Here's how the part is built. I have some questions about the finished solid (model axes, mm). Round coordinates to 2 decimals unless told otherwise and drop trailing zeros. Order: outer loops, then holes, each group sorted by start corner. A loop starts at its lowest first (then second) coordinate and runs counter-clockwise, first axis right, second up.
```python
from build123d import *

# Parameters (mm, degrees)
SKETCH1_R           = 20.32
BOSS_EXTRUDE2_DEPTH = 70.1


with BuildPart() as part:
    # Sketch1 → Boss-Extrude2 (new body)
    with BuildSketch(Plane.XY):
        with Locations((5.436965925, 8.875)):
            Circle(SKETCH1_R)
        with BuildLine():
            ThreePointArc((8.106562975, 3.61237619), (8.680765272, 1.846602096), (8.875, 0))
            ThreePointArc((8.875, 0), (-6.021266525, -6.519967365), (-0.704712549, 8.84697718))
            ThreePointArc((-0.704712549, 8.84697718), (-6.013906314, 24.19612946), (8.8646, 17.683521379))
            ThreePointArc((8.8646, 17.683521379), (8.683960375, 15.903081724), (8.149403519, 14.195204385))
            ThreePointArc((8.149403519, 14.195204385), (18.04408912, 17.284412427), (24.1046, 8.875))
            ThreePointArc((24.1046, 8.875), (18.010024125, 0.454305284), (8.106562975, 3.61237619))
        make_face(mode=Mode.SUBTRACT)
    extrude(amount=BOSS_EXTRUDE2_DEPTH)


solid = part.part
```
1) If we section it at A-A (x = 13.5): Write out the boundary of the cut face in (y, z), plus the area to 3 significant figures.
2) I'm going to push flat-ended pins straight in: pin 1 (5 mm diameter, centred on x = -7.5, z = 20, fed in from -Y); pin 2 (5 mm diameter, centred on y = 4, z = 54.5, fed in from -X); pin 3 (4 mm diameter, centred on x = 18.5, z = 17, fed in from -Y). Where does each tip first touch, or does it pass through?
3) If we section it at D-D (x = -8): Write out the boundary of the cut face in (y, z) (3 decimals), plus the area to 3 significant figures.
4) If we section it at C-C (z = 13.5): Write out the boundary of the cut face in (x, y) (3 decimals), plus the area to 3 significant figures.
5) If we section it at B-B (y = 8): Write out the boundary of the cut face in (x, z), plus the area to 3 significant figures.
6) I need wall thicknesses on line 1 (X direction, y = 17, z = 26.5); line 2 (Y direction, x = 0, z = 32.5) (3 decimals); line 3 (X direction, y = 14, z = 32). Which ranges of each line are inside material? Lowest first, please.
Solutions:
1. outline: (-9.78, 0) - (0.18, 0) - (0.18, 70.1) - (-9.78, 70.1) - close; (17.57, 0) - (27.53, 0) - (27.53, 70.1) - (17.57, 70.1) - close
1. area: 1,400 mm2
2. pin 1: stops at y = -8.56
2. pin 2: stops at x = -14.74
2. pin 3: stops at y = -8.17
3. outline: (-6.368, 0) - (-3.843, 0) - (-3.843, 70.1) - (-6.368, 70.1) - close; (3.843, 0) - (13.865, 0) - (13.865, 70.1) - (3.843, 70.1) - close; (21.502, 0) - (24.118, 0) - (24.118, 70.1) - (21.502, 70.1) - close
3. area: 1,060 mm2
4. outline: circle Ø40.64 at (5.437, 8.875); hole (-0.705, 8.847) arc R8.875 ccw (long way) to (8.107, 3.612) arc R8.865 ccw (long way) to (8.149, 14.195) arc R8.865 ccw (long way) to start
4. area: 545 mm2
5. outline: (-14.86, 0) - (-3.84, 0) - (-3.84, 70.1) - (-14.86, 70.1) - close; (24.06, 0) - (25.74, 0) - (25.74, 70.1) - (24.06, 70.1) - close
5. area: 890 mm2
6. line 1: x = -13.19 to -8.84, 8.84 to 11.7, 18.78 to 24.06
6. line 2: y = -10.704 to -8.875, 26.548 to 28.454
6. line 3: x = -14.23 to -8.06, 22.47 to 25.1
